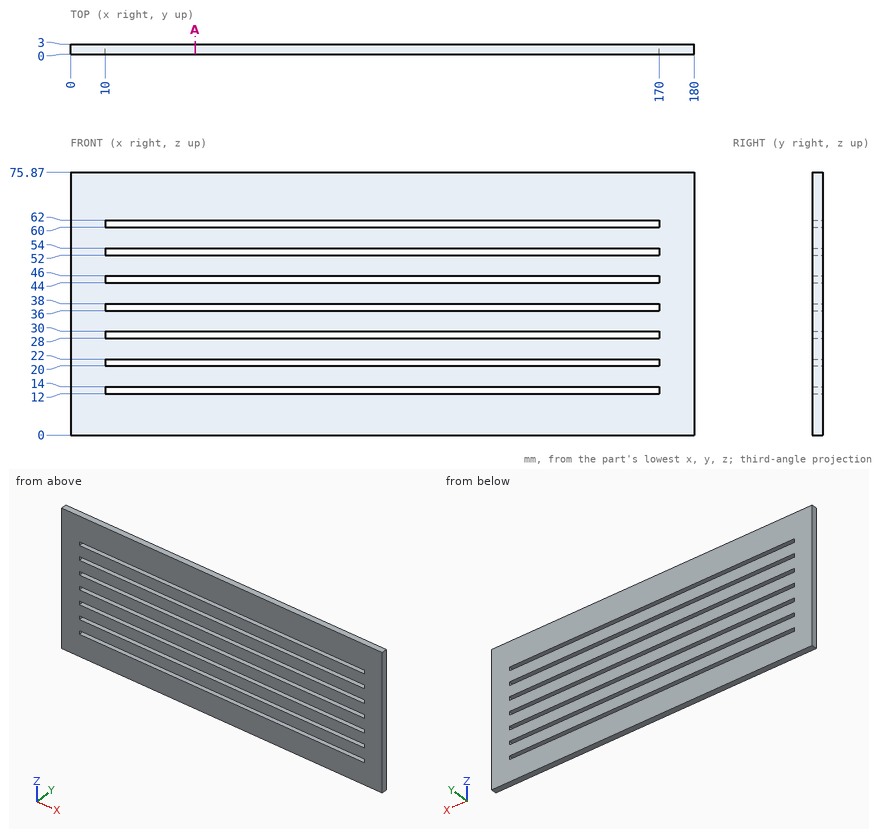
Can you work these out from the drawing? Everything is in mm from the part's minimum corner. Coordinates: 2 decimals unless noted, no trailing zeros. Write item = value, one per line.
(1) If I drill on probe 1 along X at (y, z) = (2.7, 28.5), over which ranges is the centre line in solid material (lowest first)?
Verdict:
probe_1 = 0 to 10, 170 to 180
(2) Imagine slicing it at A-A (x = 36). State how many separate pieces and enclosed holes the cut face has, and give its area (3 significant figures).
Verdict:
separate_pieces = 8
enclosed_holes = 0
area = 186 mm^2
(3) For pin 1 (1.6 mm diameter, centred on y = 1, z = 61, fed in from -X), with a flat end and sliding along its axis, tell me the tip position at first contact or that it passes through.
Verdict:
pin_1 = 0
